```python
from build123d import *

# Parameters (mm, degrees)
SKETCH_R           = 9
PAD_DEPTH          = 9
SKETCH001_W        = 2.89
SKETCH001_H        = 7
SKETCH002_R        = 2.5
POCKET_DEPTH       = 9.001
POCKET001_DEPTH    = 7
POLARPATTERN_COUNT = 20


with BuildPart() as part:
    # Sketch → Pad (new body)
    with BuildSketch(Plane.XY):
        Circle(SKETCH_R)
    extrude(amount=PAD_DEPTH)

    # Sketch001 → Groove (revolve, cut)
    with BuildSketch(Plane.XZ):
        with Locations((7.555, 4.5)):
            Rectangle(SKETCH001_W, SKETCH001_H)
    revolve(axis=Axis((0, 0, 0), (0, 0, 1)), mode=Mode.SUBTRACT)

    # Sketch002 (on Face7 of Groove) → Pocket (cut, through all)
    with BuildSketch(Plane.XY.offset(9)):
        Circle(SKETCH002_R)
    extrude(amount=-POCKET_DEPTH, mode=Mode.SUBTRACT)

    # Sketch003 (on Face3 of Groove) → Pocket001 (cut)
    with BuildSketch(Plane.XY.offset(1)):
        with BuildLine():
            ThreePointArc((6.089542, 0.499581), (5.61, 0), (6.089542, -0.499581))
            ThreePointArc((6.089542, -0.499581), (6.11, 0), (6.089542, 0.499581))
        make_face()
    pocket001 = extrude(amount=POCKET001_DEPTH, mode=Mode.SUBTRACT)

    # PolarPattern: Pocket001 ×20 about axis
    polarpattern_axis = Axis((0, 0, 1), (0, 0, 1))
    for i in range(1, POLARPATTERN_COUNT):
        add(pocket001.rotate(polarpattern_axis, i * 360 / POLARPATTERN_COUNT), mode=Mode.SUBTRACT)


solid = part.part
```
The listing builds one solid part. Answer for the finished solid, in the listing's coordinates (mm). A direction names the side the tool comes from. Coordinates: 2 decimals unless noted, no trailing zeros. Write each loop counter-clockwise with the first axis right and the second up, starting at its lowest first coordinate (ties: lowest second). Pieces come first, ordered by that corner, then holes. Notation, with made-up numbers: (-9.5, -40) -> (17.5, -40) arc R20 cw to (17.5, -23) -> close; hole circle Ø3 at (69.5, -27.75). An arc over 180 degrees is marked (long way). Write each question's results on one line, items separated by ' | '. Start each with the question number.
1) For a pull along X with two mould halves and no side action, classify faces 1 (the cylindrical face through (-5.61, -0.01, 4.45)), 2 (the cylindrical face through (-1.72, -5.34, 4.45)), 3 (the cylindrical face through (0.962, 6.034, 4.549)), 4 (the cylindrical face through (5.34, -1.72, 4.45)) as +X half, -X half, draft (parallel to the pull), parting line (faces both ways), or undercut.
2) A tool of negligible diameter and unlimited length cuts with its end or side. For faces 5 (the cylindrical face through (0.949, -6.036, 4.549)), 6 (the cylindrical face through (-0.01, 5.61, 4.45)), 7 (the cylindrical face through (6.036, 0.949, 4.549)), 8 (the cylindrical face through (3.31, -4.53, 4.45)), from which of +Z, -Z, +X, -X, +Y, -Y can it reach the whole face along a straight path? Write none if from no direction.
3) Flat-ended cylindrical pins translate along their axes: pin 1 Ø4 at (x, z) = (2, 2) entering from -Y; pin 2 Ø4 at (x, z) = (-4, 6.5) entering from -Y. Find the tip coordinate at first contact, or state that the pin passes through.
4) A cutting plane is placed at A-A (y = 0). Determine the outline of the cut face in (x, z).
5) A cutting plane is placed at D-D (y = 5). Determine the outline of the cut face in (x, z).
6) Straight lines are drawn through the part: probe 1 along Z at (x, y) = (-4.75, 7.25); probe 2 along Y at (x, z) = (-4.5, 6.25); probe 3 along X at (y, z) = (1.5, 1.5). For each, find the intervals that lie inside material, in ascending order.
7) A cutting plane is placed at C-C (x = -6.5). Determine the outline of the cut face in (y, z), then the cut area to 3 significant figures.
Values follow:
1) face 1: -X half | face 2: undercut | face 3: +X half | face 4: undercut
2) face 5: +X, -Y | face 6: +Y | face 7: +X, +Y | face 8: none
3) pin 1: y = -9 | pin 2: y = -8.59
4) outline: (-9, 0) -> (-2.5, 0) -> (-2.5, 9) -> (-9, 9) -> (-9, 8) -> (-5.61, 8) -> (-5.61, 1) -> (-9, 1) -> close; (2.5, 0) -> (9, 0) -> (9, 1) -> (5.61, 1) -> (5.61, 8) -> (9, 8) -> (9, 9) -> (2.5, 9) -> close
5) outline: (-7.48, 0) -> (7.48, 0) -> (7.48, 1) -> (3.09, 1) -> (3.09, 8) -> (7.48, 8) -> (7.48, 9) -> (-7.48, 9) -> (-7.48, 8) -> (-3.09, 8) -> (-3.09, 1) -> (-7.48, 1) -> close
6) probe 1: 0 to 1, 8 to 9 | probe 2: -4.13 to -3.82, -3.36 to 3.36, 3.82 to 4.13 | probe 3: -5.5 to -2, 2 to 5.5
7) outline: (-6.22, 0) -> (6.22, 0) -> (6.22, 1) -> (-6.22, 1) -> close; (-6.22, 8) -> (6.22, 8) -> (6.22, 9) -> (-6.22, 9) -> close | area: 24.9 mm²
